For this review, take the finished solid that the model builds, in its own axes (mm). Face numbers are marked on the shaded views. A direction names the side the tool comes from. Give positions to 0.01 mm unless a question says otherwise; leave off trailing zeros. Order: outer loops, then holes, each group sorted by start corner. A loop starts at its lowest first (then second) coordinate and runs counter-clockwise, first axis right, second up. Notation, with made-up numbers: (40, 55.5) -> (91, 55.5) arc R15 ccw to (91, 75.5) -> close; hole circle Ø9 at (-36, 33.5). An arc over 180 degrees is marked (long way). One line per item, written item: value. Start each with the question number.
from build123d import *

# Parameters (mm, degrees)
F1_DEPTH = 36
F2_DEPTH = 16
F3_SIZE  = 0.6


with BuildPart() as f1:
    # F0 (on Top) → F1 (new body)
    with BuildSketch(Plane.XY):
        Polygon((-7.451849, -0.85), (7.451849, -0.85), (10, -0.85), (17.7, -0.85), (17.7, 0.85), (-17.7, 0.85), (-17.7, -0.85), (-10, -0.85), align=None)
    extrude(amount=F1_DEPTH)

    # F0 (on Top) → F2 (join)
    with BuildSketch(Plane.XY):
        with BuildLine():
            ThreePointArc((-4, -8.45), (-3.813206, -7.241918), (-3.270269, -6.146668))
            Line((-3.270269, -6.146668), (-7.451849, -0.85))
            Line((-7.451849, -0.85), (-10, -0.85))
            Line((-10, -0.85), (-4, -8.45))
        make_face()
        with BuildLine():
            Line((7.451849, -0.85), (3.270269, -6.146668))
            ThreePointArc((3.270269, -6.146668), (3.813206, -7.241918), (4, -8.45))
            Line((4, -8.45), (10, -0.85))
            Line((10, -0.85), (7.451849, -0.85))
        make_face()
        with BuildLine():
            ThreePointArc((-1.987411, -7.771621), (0, -6.35), (1.987411, -7.771621))
            Line((1.987411, -7.771621), (3.270269, -6.146668))
            ThreePointArc((3.270269, -6.146668), (0, -4.45), (-3.270269, -6.146668))
            Line((-3.270269, -6.146668), (-1.987411, -7.771621))
        make_face()
        with BuildLine():
            ThreePointArc((1.987411, -7.771621), (2.071662, -8.106171), (2.1, -8.45))
            ThreePointArc((2.1, -8.45), (-0.343829, -10.521662), (-1.987411, -7.771621))
            Line((-1.987411, -7.771621), (-3.270269, -6.146668))
            ThreePointArc((-3.270269, -6.146668), (-3.813206, -7.241918), (-4, -8.45))
            ThreePointArc((-4, -8.45), (0, -12.45), (4, -8.45))
            ThreePointArc((4, -8.45), (3.813206, -7.241918), (3.270269, -6.146668))
            Line((3.270269, -6.146668), (1.987411, -7.771621))
        make_face()
    extrude(amount=F2_DEPTH)

    # F3
    f3_edges = [f1.edges().sort_by_distance(p)[0] for p in [
        (1.987411, -9.128379, 0),
        (1.987411, -9.128379, 16),
    ]]
    chamfer(f3_edges, length=F3_SIZE)


solid = f1.part
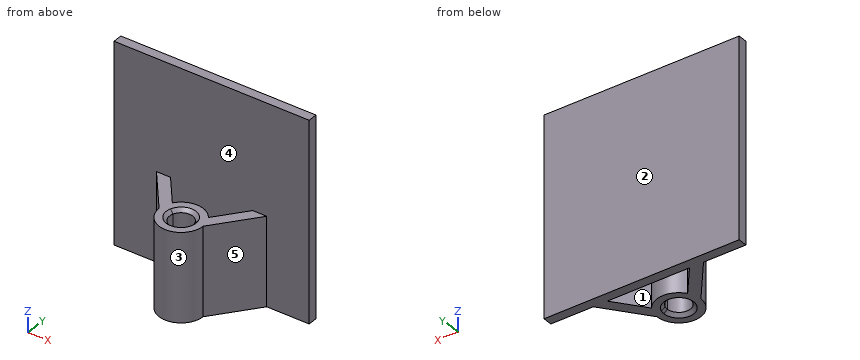
Q1. For the marked faces 1 and 2, list the 3-axis set-ups (+Z, -Z, +X, -X, +Y, -Y) from which the entire face can be reached by the end or side of a thin tool; tool diameter is ignored.
Q2. Take a section at C-C (y = -3). State the section outline as (x, z) points, and give its area (3 significant figures).
Q3. Mouldability with a two-part tool opening along X and no side actions: class the marked faces 3, 4 and 5 as pulls with the +X half, pulls with the -X half, needs draft (parallel to the pull), parting line crosses it, or undercut.
Q4. For pin 1 Ø4 at (y, z) = (-2, 20) entering from -X; pin 2 Ø3 at (x, y) = (9, -5) entering from +Z; pin 3 Ø5 at (y, z) = (-5.5, 11) entering from -X; pin 4 Ø2 at (x, y) = (1.5, -5) entering from +Z, all flat-tipped, find the tip position at first contact; note any pin that passes through.
Q5. Take a section at A-A (x = 0). State the section outline as (y, z) points.
Q6. Take a section at D-D (y = -5). State the section outline as (x, z) points.
Q7. For line 1 along Y through (x, z) = (0, 10.25); line 2 along X through (y, z) = (-8.45, 9); line 3 along Y through (x, z) = (-6.5, 33), list the stretches that pass through material, from the lowest coordinate up.
Q8. Take a section at B-B (z = 14.5). State the section outline as (x, y) points.
Answers below:
1. face 1: +Z, -Z
1. face 2: +Z, -Z, +X, -X, +Y
2. outline: (-8.3, 0) -> (-5.75, 0) -> (-5.75, 16) -> (-8.3, 16) -> close; (5.75, 0) -> (8.3, 0) -> (8.3, 16) -> (5.75, 16) -> close
2. area: 81.5 mm²
3. face 3: parting line crosses it
3. face 4: undercut
3. face 5: pulls with the +X half
4. pin 1: stops at x = -17.7
4. pin 2: passes through
4. pin 3: stops at x = -8.3
4. pin 4: stops at z = 16
5. outline: (-12.45, 0) -> (-11.15, 0) -> (-10.55, 0.6) -> (-10.55, 15.4) -> (-11.15, 16) -> (-12.45, 16) -> close; (-6.35, 0.6) -> (-5.75, 0) -> (-4.45, 0) -> (-4.45, 16) -> (-5.75, 16) -> (-6.35, 15.4) -> close; (-0.85, 0) -> (0.85, 0) -> (0.85, 36) -> (-0.85, 36) -> close
6. outline: (-6.72, 0) -> (-4.18, 0) -> (-4.18, 16) -> (-6.72, 16) -> close; (-2.02, 0) -> (2.02, 0) -> (2.02, 16) -> (-2.02, 16) -> close; (4.18, 0) -> (6.72, 0) -> (6.72, 16) -> (4.18, 16) -> close
7. line 1: y = -12.45 to -10.55, -6.35 to -4.45, -0.85 to 0.85
7. line 2: x = -4 to -2.1, 2.1 to 4
7. line 3: y = -0.85 to 0.85
8. outline: (-17.7, -0.85) -> (-10, -0.85) -> (-4, -8.45) arc R4 ccw to (4, -8.45) -> (10, -0.85) -> (17.7, -0.85) -> (17.7, 0.85) -> (-17.7, 0.85) -> close; hole (-7.45, -0.85) -> (-3.27, -6.15) arc R4 cw to (3.27, -6.15) -> (7.45, -0.85) -> close; hole (1.99, -7.77) arc R2.1 ccw (long way) to (2.1, -8.45) arc R2.1 ccw to start
